CAD build for the part. Positions are in the model's coordinates, mm. Give positions to 0.01 mm unless a question says otherwise; leave off trailing zeros. Loops run counter-clockwise (first coordinate to the right, second up) from the corner with the lowest first, then second, coordinate; pieces in that order, holes last.
```python
from build123d import *

# Parameters (mm, degrees)
CHAMFER1_SIZE   = 0.359317173
CHAMFER1_SIZE_2 = 0.5


with BuildPart() as part:
    # Sketch2 → Revolve1 (revolve)
    with BuildSketch(Plane.XY):
        with BuildLine():
            Line((-9.525, -4.5), (-9.525, 4.5))
            Line((-9.525, 4.5), (-6.493073232, 4.5))
            ThreePointArc((-6.493073232, 4.5), (-7.9, 0), (-6.493073232, -4.5))
            Line((-6.493073232, -4.5), (-9.525, -4.5))
        make_face()
    revolve(axis=Axis((0, -4.5, 0), (0, 1, 0)))

    # Chamfer1
    # the kernel refuses this chamfer: 0.5, 0.359317173 mm, written as the material it takes off along each edge
    with BuildSketch(Plane(origin=(0, 4.5, 0), x_dir=(-1, 0, 0), z_dir=(0, 0, -1))) as chamfer1_piece_1:
        with BuildLine():
            Line((6.493073232 + CHAMFER1_SIZE, 0), (6.773611969, -0.434513449))
            ThreePointArc((6.773611969, -0.434513449), (6.640861095, -0.221102487), (6.493073232, 0))
            Line((6.493073232, 0), (6.493073232 + CHAMFER1_SIZE, 0))
        make_face()
    revolve(axis=Axis((0, 4.5, 0), (0, 1, 0)), mode=Mode.SUBTRACT)
    with BuildSketch(Plane(origin=(0, 4.5, 0), x_dir=(-1, 0, 0), z_dir=(0, 0, -1))) as chamfer1_piece_2:
        Polygon((9.525, -CHAMFER1_SIZE_2), (9.525 - CHAMFER1_SIZE_2, 0), (9.525, 0), align=None)
    revolve(axis=Axis((0, 4.5, 0), (0, 1, 0)), mode=Mode.SUBTRACT)
    with BuildSketch(Plane(origin=(0, -4.5, 0), x_dir=(-1, 0, 0), z_dir=(0, 0, -1))) as chamfer1_piece_3:
        Polygon((9.525 - CHAMFER1_SIZE_2, 0), (9.525, CHAMFER1_SIZE_2), (9.525, 0), align=None)
    revolve(axis=Axis((0, -4.5, 0), (0, 1, 0)), mode=Mode.SUBTRACT)
    with BuildSketch(Plane(origin=(0, -4.5, 0), x_dir=(-1, 0, 0), z_dir=(0, 0, -1))) as chamfer1_piece_4:
        with BuildLine():
            Line((6.493073232 + CHAMFER1_SIZE_2, 0), (6.691823244, 0.301249988))
            ThreePointArc((6.691823244, 0.301249988), (6.595276141, 0.151168821), (6.493073232, 0))
            Line((6.493073232, 0), (6.493073232 + CHAMFER1_SIZE_2, 0))
        make_face()
    revolve(axis=Axis((0, -4.5, 0), (0, 1, 0)), mode=Mode.SUBTRACT)


solid = part.part
```
1. Saw through at B-B, the plane x = 0. List the corners of the cut face in (y, z) (3 decimals).
Responses:
outline: (-4.5, -9.025) - (-4, -9.525) - (4, -9.525) - (4.5, -9.025) - (4.5, -6.852) - (4.065, -6.774) arc R7.9 cw to (-4.199, -6.692) - (-4.5, -6.993) - close; (-4.5, 6.993) - (-4.199, 6.692) arc R7.9 cw to (4.065, 6.774) - (4.5, 6.852) - (4.5, 9.025) - (4, 9.525) - (-4, 9.525) - (-4.5, 9.025) - close
2. Drop flat-ended pins along their axis: pin 1 (1 mm diameter, centred on x = -5, z = -3, fed in from +Y); pin 2 (1 mm diameter, centred on y = 2.5, z = 2.5, fed in from -X); pin 3 (1.5 mm diameter, centred on y = -2, z = 1.5, fed in from -X); pin 4 (5 mm diameter, centred on x = -3.5, y = 0.5, fed in from -Z). Give the stop position or say it passes through.
Responses:
pin 1: passes through
pin 2: stops at x = -9.31
pin 3: stops at x = -9.5
pin 4: stops at z = -9.47
3. Saw through at A-A, the plane z = 0. List the corners of the cut face in (x, y) (3 decimals).
Responses:
outline: (-9.525, -4) - (-9.025, -4.5) - (-6.993, -4.5) - (-6.692, -4.199) arc R7.9 cw to (-6.774, 4.065) - (-6.852, 4.5) - (-9.025, 4.5) - (-9.525, 4) - close; (6.692, -4.199) - (6.993, -4.5) - (9.025, -4.5) - (9.525, -4) - (9.525, 4) - (9.025, 4.5) - (6.852, 4.5) - (6.774, 4.065) arc R7.9 cw to start
4. Saw through at D-D, the plane y = 2.5. List the corners of the cut face in (x, z) (3 decimals).
Responses:
outline: circle Ø19.05 at (0, 0); hole circle Ø14.988 at (0, 0)
5. Saw through at C-C, the plane y = -0.5. List the corners of the cut face in (x, z) (3 decimals).
Responses:
outline: circle Ø19.05 at (0, 0); hole circle Ø15.768 at (0, 0)
6. Probe line 1 along Z through (x, y) = (-7.25, 0.5); line 2 along Z through (x, y) = (0.5, 3); line 3 along X through (y, z) = (-3.5, -5.75). List the from-to ranges inside material, lowest first.
Responses:
line 1: z = -6.18 to -3.1, 3.1 to 6.18
line 2: z = -9.51 to -7.29, 7.29 to 9.51
line 3: x = -7.59 to -4.13, 4.13 to 7.59
7. Pull direction X, two halves, no side cores. Call faces 1 (the face through (7.559, 0.056, -5.796)), 2 (the face through (1, 4.5, 7)): released by +X, released by -X, zero draft, split by the parting line, or undercut.
Responses:
face 1: split by the parting line
face 2: zero draft
